Source: CAD feature listing. Evaluate the final solid. Frame: model axes, mm. A direction names the side the tool comes from. Give positions to 0.01 mm unless a question says otherwise; leave off trailing zeros. Order: outer loops, then holes, each group sorted by start corner. A loop starts at its lowest first (then second) coordinate and runs counter-clockwise, first axis right, second up. Notation, with made-up numbers: M 5,46.5 L 14,46.5 A18 ccw 14,59.5 Z; hole C 20.25,41 d1. An arc over 180 degrees is marked long. Answer as a JSON object with one key per item and string values. Group by question number.
1. Material intervals for L1, parallel to Y at x = -1.5, z = 0; L2, parallel to Y at x = -2, z = -2.5; L3, parallel to Y at x = 4.25, z = -0.25, sorted ascending. Write a range as [from, to].
2. Section query D-D (y = 52). Output: boundary loops of the cut face in (x, z) (1 decimal), plus the area to 3 significant figures.
3. Pin query (flat end, axial travel): P1, Ø1.5, axis at x = 2, y = 34, coming from the +Z side; P2, Ø4, axis at x = 3, y = 51.5, coming from the -Z side; P3, Ø1.5, axis at x = 1, z = -1, coming from the -Y side. Return the tip coordinate at first contact, or that it passes through.
4. Pull-direction query (Z, two-part tool) for faces 3 (the flat face through (0, 65, 0)), 4 (the cylindrical face through (-3.373, 11.586, -0.113)), 5 (the cylindrical face through (1.37, 32.04, 4.35)); classes: +Z half, -Z half, draft (parallel to the pull), parting line (faces both ways), or undercut.
5. Set-up query: faces 1 (the flat face through (3, 0, 0)), 2 (the flat face through (2.456, 12, 0)). Return all of +Z, -Z, +X, -X, +Y, -Y with unobstructed straight access to the full face (end or side cutting, diameter ignored); none if empty.
from build123d import *

# Parameters (mm, degrees)
SKETCH1_R               = 4.5625
BOSS_EXTRUDE1_DEPTH     = 65
CUT_EXTRUDE1_DEPTH      = 66.319467332
CUT_EXTRUDE1_DEPTH_BACK = 66.319467332
SKETCH2_R               = 1.75
CUT_EXTRUDE2_DEPTH      = 23.5


with BuildPart() as part:
    # Sketch1 → Boss-Extrude1 (new body)
    with BuildSketch(Plane(origin=(0, 0, 0), x_dir=(1, 0, 0), z_dir=(0, 1, 0))):
        with Locations(Location((0, 0, 0), (0, 0, 270))):
            Circle(SKETCH1_R)
    extrude(amount=BOSS_EXTRUDE1_DEPTH)

    # Sketch2 → Cut-Extrude1 (cut, two sides: drawn at the far end of the back side and taken through both)
    with BuildSketch(Plane(origin=(0, 0, 0), x_dir=(0, 0, -1), z_dir=(1, 0, 0)).offset(-CUT_EXTRUDE1_DEPTH_BACK)):
        with Locations((0, 32.5)):
            Circle(SKETCH2_R)
    extrude(amount=CUT_EXTRUDE1_DEPTH + CUT_EXTRUDE1_DEPTH_BACK, mode=Mode.SUBTRACT)

    # Sketch4 → Cut-Extrude2 (cut)
    with BuildSketch(Plane(origin=(0, 0, 0), x_dir=(-1, 0, 0), z_dir=(0, -1, 0))):
        with BuildLine():
            Line((-2.455890877, -2.315), (-2.455890877, 2.315))
            ThreePointArc((-2.455890877, 2.315), (3.375, 0), (-2.455890877, -2.315))
        make_face()
    extrude(amount=-CUT_EXTRUDE2_DEPTH, mode=Mode.SUBTRACT)


solid = part.part
Answer sheet:
{
 "1": {"L1": "[23.5, 30.75], [34.25, 65]", "L2": "[23.5, 65]", "L3": "[0, 30.77], [34.23, 65]"},
 "2": {"outline": "C 0,0 d9.1", "area": "65.4 mm^2"},
 "3": {"P1": "z = 4.39", "P2": "z = -4.45", "P3": "y = 23.5"},
 "4": {"face 3": "draft", "face 4": "undercut", "face 5": "parting line"},
 "5": {"face 1": "+Z, -Z, +X, -X, -Y", "face 2": "-Y"}
}
